from build123d import *

# Parameters (mm, degrees)
SKETCH1_W           = 70
SKETCH1_H           = 70
BOSS_EXTRUDE1_DEPTH = 2
SKETCH2_W           = 2
SKETCH2_H           = 20
SKETCH2_W_2         = 20
SKETCH2_H_2         = 2
CUT_EXTRUDE1_DEPTH  = 2
CUT_EXTRUDE2_DEPTH  = 10


with BuildPart() as part:
    # Sketch1 → Boss-Extrude1 (new body)
    with BuildSketch(Plane.XY):
        Rectangle(SKETCH1_W, SKETCH1_H)
    extrude(amount=-BOSS_EXTRUDE1_DEPTH)

    # Sketch2 → Cut-Extrude1 (cut)
    with BuildSketch(Plane.XY):
        with Locations((-34, 15)):
            Rectangle(SKETCH2_W, SKETCH2_H)
        with Locations((-34, -15)):
            Rectangle(SKETCH2_W, SKETCH2_H)
        with Locations((-15, -34)):
            Rectangle(SKETCH2_W_2, SKETCH2_H_2)
        with Locations((15, -34)):
            Rectangle(SKETCH2_W_2, SKETCH2_H_2)
        with Locations((34, -15)):
            Rectangle(SKETCH2_W, SKETCH2_H)
        with Locations((34, 15)):
            Rectangle(SKETCH2_W, SKETCH2_H)
        with Locations((15, 34)):
            Rectangle(SKETCH2_W_2, SKETCH2_H_2)
        with Locations((-15, 34)):
            Rectangle(SKETCH2_W_2, SKETCH2_H_2)
    extrude(amount=-CUT_EXTRUDE1_DEPTH, mode=Mode.SUBTRACT)

    # Sketch6 → Cut-Extrude2 (cut)
    with BuildSketch(Plane(origin=(0, 0, -2), x_dir=(-1, 0, 0), z_dir=(0, 0, -1))):
        Polygon((-9.325, -14.5), (-9.325, -22.5), (9.325, -22.5), (9.325, -14.5), (17.325, -14.5), (17.325, 14.5), (9.325, 14.5), (9.325, 22.5), (-9.325, 22.5), (-9.325, 14.5), (-17.325, 14.5), (-17.325, -14.5), align=None)
        with BuildLine():
            Line((-9.325, 22.5), (-9.325, 14.5))
            Line((-9.325, 14.5), (-17.325, 14.5))
            ThreePointArc((-17.325, 14.5), (-14.981854249, 20.156854249), (-9.325, 22.5))
        make_face()
        with BuildLine():
            ThreePointArc((9.325, 22.5), (14.981854249, 20.156854249), (17.325, 14.5))
            Line((17.325, 14.5), (9.325, 14.5))
            Line((9.325, 14.5), (9.325, 22.5))
        make_face()
        with BuildLine():
            ThreePointArc((-9.325, -22.5), (-14.981854249, -20.156854249), (-17.325, -14.5))
            Line((-17.325, -14.5), (-9.325, -14.5))
            Line((-9.325, -14.5), (-9.325, -22.5))
        make_face()
        with BuildLine():
            Line((9.325, -22.5), (9.325, -14.5))
            Line((9.325, -14.5), (17.325, -14.5))
            ThreePointArc((17.325, -14.5), (14.981854249, -20.156854249), (9.325, -22.5))
        make_face()
    extrude(amount=-CUT_EXTRUDE2_DEPTH, mode=Mode.SUBTRACT)


solid = part.part
Input: part model. Units: mm. Frame: model coordinates. A direction names the side the tool comes from. Coordinates: 2 decimals unless noted, no trailing zeros. Loops run counter-clockwise (first coordinate to the right, second up) from the corner with the lowest first, then second, coordinate; pieces in that order, holes last.
Q1. Contact query for a flat-ended pin moving along its axis: pin 1 (0.6 mm diameter, centred on x = -16, z = -1, fed in from +Y). Output: stop coordinate, or through.
Q2. Draft query along Y for faces 5 (the face through (-15, 33, -1)), 6 (the face through (5, -34, -1)), 7 (the face through (-33, -15, -1)). Return one class per face: +Y half, -Y half, draft (parallel to the pull), parting line (faces both ways), or undercut.
Q3. Cut plane B-B (y = 20). Output: boundary loops of the cut face in (x, z).
Q4. Set-up query: faces 1 (the face through (-5, -34, -1)), 2 (the face through (34, 5, -1)), 3 (the face through (-17.325, 0, -1)), 4 (the face through (-33, 15, -1)). Return all of +Z, -Z, +X, -X, +Y, -Y with unobstructed straight access to the full face (end or side cutting, diameter ignored); none if empty.
Q5. Cut plane A-A (x = 0). Output: boundary loops of the cut face in (y, z), then the cut area to 3 significant figures.
Q6. Material intervals for line 1 (X direction, y = -2.5, z = -1.35) (3 decimals); line 2 (X direction, y = 10, z = -0.5) (3 decimals); line 3 (Y direction, x = -5.5, z = -0.5), sorted ascending.
Working result:
1. pin 1: stops at y = 33
2. face 5: +Y half
2. face 6: draft
2. face 7: undercut
3. outline: (-33, -2) - (-15.13, -2) - (-15.13, 0) - (-33, 0) - close; (15.13, -2) - (33, -2) - (33, 0) - (15.13, 0) - close
4. face 1: +Z, -Z, -Y
4. face 2: +Z, -Z, +X
4. face 3: +Z, -Z
4. face 4: +Z, -Z, -X
5. outline: (-35, -2) - (-22.5, -2) - (-22.5, 0) - (-35, 0) - close; (22.5, -2) - (35, -2) - (35, 0) - (22.5, 0) - close
5. area: 50.0 mm2
6. line 1: x = -35 to -17.325, 17.325 to 35
6. line 2: x = -33 to -17.325, 17.325 to 33
6. line 3: y = -33 to -22.5, 22.5 to 33
